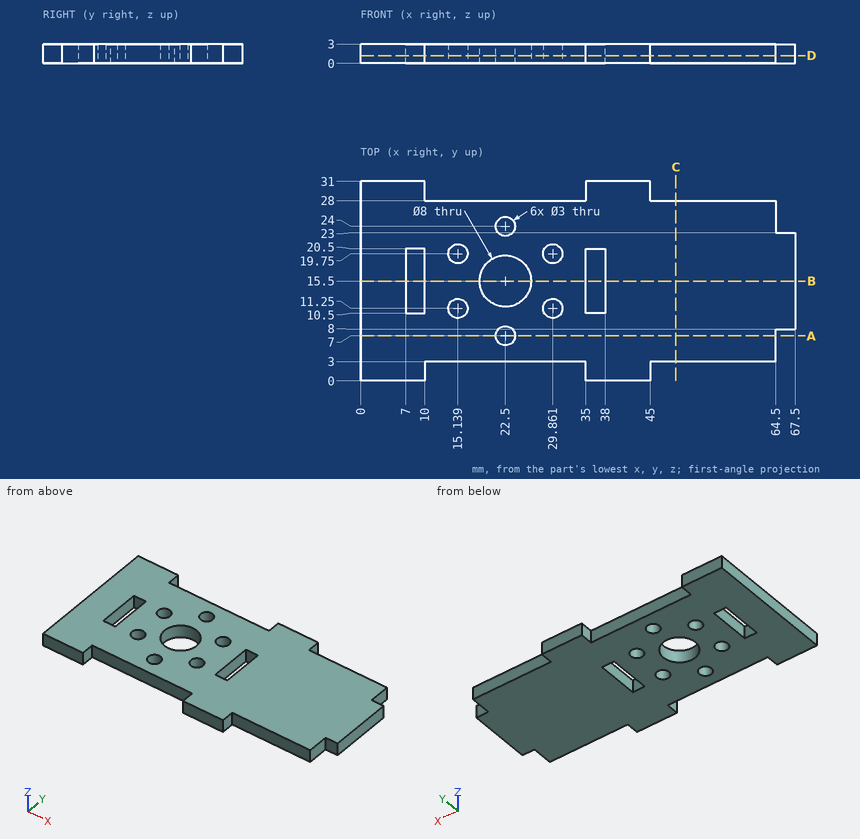
Study the drawing (mm; zero at the part's minimum x, y, z) and answer. Give positions to 0.01 mm unless a question says otherwise; leave off trailing zeros. Write each loop counter-clockwise with the first axis right and the second up, starting at its lowest first coordinate (ties: lowest second). Pieces come first, ordered by that corner, then holes. Notation, with made-up numbers: (15, 21.5) -> (28, 21.5) arc R29 ccw to (28, 58.5) -> close; hole circle Ø7 at (54, 83). An arc over 180 degrees is marked (long way). Answer in a Markdown table with one row per item.
1) Section C-C on x = 49 is taken. Give the vertices of the cut face in (y, z), plus the area to 3 significant figures.
Results list:
| item | result |
|---|---|
| outline | (3, 0) -> (28, 0) -> (28, 3) -> (3, 3) -> close |
| area | 75.0 mm^2 |
2) Each of these flat-tipped pins is pushed along its axis until it touches: pin 1 Ø0.9 at (y, z) = (26, 2) entering from +X; pin 2 Ø1 at (x, z) = (16.5, 2.5) entering from +Y. Where does it stop, or does it pass through?
Results list:
| item | result |
|---|---|
| pin 1 | x = 64.5 |
| pin 2 | y = 28 |
3) Section A-A on y = 7 is taken. Give the vertices of the cut face in (x, z).
Results list:
| item | result |
|---|---|
| outline | (0, 0) -> (21, 0) -> (21, 3) -> (0, 3) -> close; (24, 0) -> (64.5, 0) -> (64.5, 3) -> (24, 3) -> close |
4) Straight lines are drawn through the part: line 1 (Y direction, x = 22.5, z = 1.35); line 2 (X direction, y = 7, z = 0.9); line 3 (Y direction, x = 57.5, z = 0.5). For each, find the intervals that lie inside material, in ascending order. Write a range as [from, to].
Results list:
| item | result |
|---|---|
| line 1 | [3, 5.5], [8.5, 11.5], [19.5, 22.5], [25.5, 28] |
| line 2 | [0, 21], [24, 64.5] |
| line 3 | [3, 28] |
5) Section D-D on z = 1.2 is taken. Count the separate pieces of the cut face and the enclosed holes in it, plus the area to 3 significant figures.
Results list:
| item | result |
|---|---|
| separate pieces | 1 |
| enclosed holes | 9 |
| area | 1,620 mm^2 |
6) Section B-B on y = 15.5 is taken. Give the vertices of the cut face in (x, z).
Results list:
| item | result |
|---|---|
| outline | (0, 0) -> (7, 0) -> (7, 3) -> (0, 3) -> close; (10, 0) -> (18.5, 0) -> (18.5, 3) -> (10, 3) -> close; (26.5, 0) -> (35, 0) -> (35, 3) -> (26.5, 3) -> close; (38, 0) -> (67.5, 0) -> (67.5, 3) -> (38, 3) -> close |
